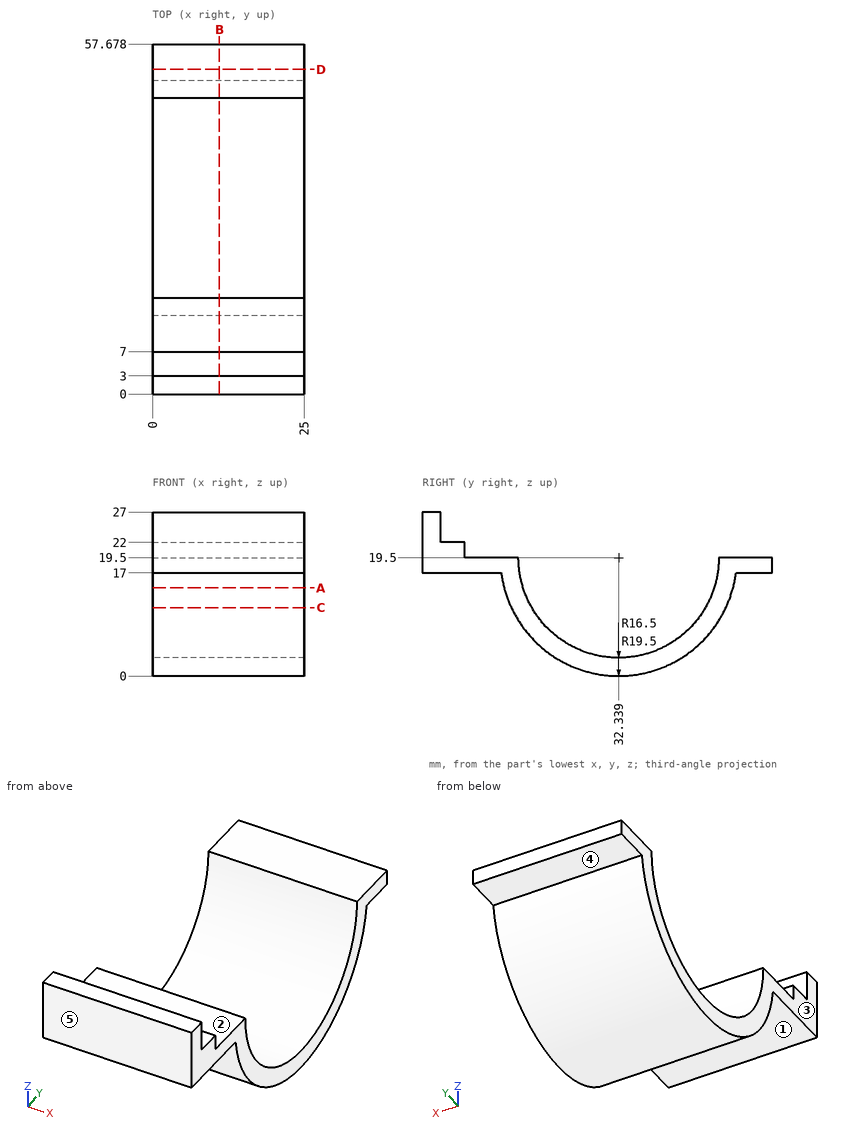
Job drawing, mm, ordinate dimensions from the low corner. One solid piece. A direction names the side the tool comes from. Coordinates: 2 decimals unless noted, no trailing zeros. Order: outer loops, then holes, each group sorted by start corner. A loop starts at its lowest first (then second) coordinate and runs counter-clockwise, first axis right, second up. Notation, with made-up numbers: (8, 30) -> (30, 30) arc R30 cw to (30, 65) -> close; hole circle Ø11 at (36.5, 22.5). An arc over 180 degrees is marked (long way). Return JSON: item names as keys, results as strings. Group by question number.
Item 1: Tool access for the marked faces 1, 2, 3, 4 and 5: list every direction of +Z, -Z, +X, -X, +Y, -Y with a clear straight run to the whole face (end or side of a thin tool).
Item 2: Saw through at C-C on z = 11.25. Write the cut outline in (x, y), then the cut area to 3 significant figures.
Item 3: Flat gauge pins, fed straight in: P1, Ø7, axis at x = 10, y = 9.5, coming from the +Z side; P2, Ø3, axis at x = 9.5, y = 56, coming from the -Z side; P3, Ø2, axis at x = 10, z = 21.5, coming from the +Y side. Where does each tip first touch, or does it go through?
Item 4: Wall check: line 1 along Z through (x, y) = (9.75, 5); line 2 along Z through (x, y) = (12.25, 9.5); line 3 along Y through (x, z) = (7, 5) (1 decimal). Give the ranges that are in metal, low to high. Write a range as [from, to].
Item 5: Saw through at A-A on z = 14.5. Write the cut outline in (x, y) (1 decimal), then the cut area to 3 significant figures.
Item 6: Saw through at B-B on x = 11. Write the cut outline in (y, z), then the cut area to 3 significant figures.
Item 7: Saw through at D-D on y = 53.5. Write the cut outline in (x, z).
Values found:
{
 "1": {"face 1": "-Z, +X, -X, -Y", "face 2": "+Z, +X, -X, +Y", "face 3": "+Z, -Z, -X, +Y, -Y", "face 4": "-Z, +X, -X, +Y", "face 5": "+Z, -Z, +X, -X, -Y"},
 "2": {"outline": "(0, 14.67) -> (25, 14.67) -> (25, 18.05) -> (0, 18.05) -> close; (0, 46.63) -> (25, 46.63) -> (25, 50.01) -> (0, 50.01) -> close", "area": "169 mm2"},
 "3": {"P1": "stops at z = 22", "P2": "stops at z = 17", "P3": "stops at y = 7"},
 "4": {"line 1": "z = [17, 22]", "line 2": "z = [17, 19.5]", "line 3": "y = [19.3, 24.5], [40.2, 45.4]"},
 "5": {"outline": "(0, 13.5) -> (25, 13.5) -> (25, 16.6) -> (0, 16.6) -> close; (0, 48.1) -> (25, 48.1) -> (25, 51.2) -> (0, 51.2) -> close", "area": "156 mm2"},
 "6": {"outline": "(0, 17) -> (13, 17) arc R19.5 ccw to (51.68, 17) -> (57.68, 17) -> (57.68, 19.5) -> (48.84, 19.5) arc R16.5 cw to (15.84, 19.5) -> (7, 19.5) -> (7, 22) -> (3, 22) -> (3, 27) -> (0, 27) -> close", "area": "249 mm2"},
 "7": {"outline": "(0, 17) -> (25, 17) -> (25, 19.5) -> (0, 19.5) -> close"}
}
